Design review of the part built by this model. Coordinates are the model's own, in mm. A direction names the side the tool comes from. Coordinates: 2 decimals unless noted, no trailing zeros. Write each loop counter-clockwise with the first axis right and the second up, starting at its lowest first coordinate (ties: lowest second). Pieces come first, ordered by that corner, then holes.
Q1. For faces 1 (the cylindrical face through (-15.02, 3.23, 0.53)), 2 (the flat face through (9.01, 3.51, -1.74)), 3 (the flat face through (-13.01, 0.99, -1.74)), list the 3-axis set-ups (+Z, -Z, +X, -X, +Y, -Y) from which the entire face can be reached by the end or side of a thin tool; tool diameter is ignored.
Q2. Take a section at B-B, the plane y = 2.9. Write out the cut boundary in (x, z).
Q3. The part is to be moulded in two halves that separate along Z. For faces 4 (the flat face through (-12, 1, 0)), 5 (the flat face through (-5, 4.5, 5)), 6 (the cylindrical face through (-17.46, 2.22, -0.52)), say which applies: released by +Z, released by -Z, zero draft, split by the parting line, or undercut.
Q4. For pin 1 Ø0.6 at (y, z) = (1, -0.5) entering from -X; pin 2 Ø1.2 at (x, z) = (9.5, 0.5) entering from +Y; pin 3 Ø1 at (y, z) = (2.5, 8) entering from +X, all flat-tipped, find the tip position at first contact; note any pin that passes through.
Q5. For L1, parallel to X at y = 1.6, z = 0; L2, parallel to X at y = 0.35, z = 0; L3, parallel to X at y = 3, z = -2.25, list the stretches that pass through material, from the lowest coordinate up.
Q6. Take a section at D-D, the plane x = -10.5. Write out the cut boundary in (y, z).
Q7. Take a section at C-C, the plane x = 0. Write out the cut boundary in (y, z), plus the area to 4 significant figures.
Q8. Take a section at A-A, the plane z = 0. Write out the cut boundary in (x, y), plus the area to 3 significant figures.
from build123d import *

# Parameters (mm, degrees)
SKETCH1_R           = 4
SKETCH1_R_2         = 1.15
BOSS_EXTRUDE1_DEPTH = 4.5
SKETCH2_R           = 6
CUT_EXTRUDE1_DEPTH  = 3.5
CUT_EXTRUDE2_DEPTH  = 2
CUT_EXTRUDE3_DEPTH  = 2


with BuildPart() as part:
    # Sketch1 → Boss-Extrude1 (new body)
    with BuildSketch(Plane(origin=(0, 0, 0), x_dir=(1, 0, 0), z_dir=(0, 1, 0))):
        with BuildLine():
            Line((3, 6.873863542), (11.4, 3.207802986))
            ThreePointArc((11.4, 3.207802986), (13.439020979, 0.650488054), (12.474873734, -2.474873734))
            Line((12.474873734, -2.474873734), (2.474873734, -12.474873734))
            ThreePointArc((2.474873734, -12.474873734), (0.28868186, -13.488074366), (-2.034333678, -12.848067149))
            Line((-2.034333678, -12.848067149), (-16.034333678, -2.848067149))
            ThreePointArc((-16.034333678, -2.848067149), (-17.452321053, 0.575742432), (-15, 3.354101966))
            Line((-15, 3.354101966), (-2.142857143, 7.187361356))
            ThreePointArc((-2.142857143, 7.187361356), (0.456337254, 7.486104215), (3, 6.873863542))
        make_face()
        with Locations(Location((0, 0, 0), (0, 0, 270))):
            Circle(SKETCH1_R, mode=Mode.SUBTRACT)
        with Locations(Location((-14, 0, 0), (0, 0, 270))):
            Circle(SKETCH1_R_2, mode=Mode.SUBTRACT)
        with Locations(Location((10, 0, 0), (0, 0, 270))):
            Circle(SKETCH1_R_2, mode=Mode.SUBTRACT)
        with Locations(Location((0, -10, 0), (0, 0, 270))):
            Circle(SKETCH1_R_2, mode=Mode.SUBTRACT)
    extrude(amount=BOSS_EXTRUDE1_DEPTH)

    # Sketch2 → Cut-Extrude1 (cut)
    with BuildSketch(Plane(origin=(0, 4.5, 0), x_dir=(1, 0, 0), z_dir=(0, 1, 0))):
        with Locations(Location((0, 0, 0), (0, 0, 270))):
            Circle(SKETCH2_R)
    extrude(amount=-CUT_EXTRUDE1_DEPTH, mode=Mode.SUBTRACT)

    # Sketch3 → Cut-Extrude2 (cut)
    with BuildSketch(Plane(origin=(0, 4.5, 0), x_dir=(1, 0, 0), z_dir=(0, 1, 0))):
        Polygon((12, -1.154700538), (12, 1.154700538), (10, 2.309401077), (8, 1.154700538), (8, -1.154700538), (10, -2.309401077), align=None)
        Polygon((2.309401077, -10), (1.154700538, -8), (-1.154700538, -8), (-2.309401077, -10), (-1.154700538, -12), (1.154700538, -12), align=None)
    extrude(amount=-CUT_EXTRUDE2_DEPTH, mode=Mode.SUBTRACT)

    # Sketch4 → Cut-Extrude3 (cut)
    with BuildSketch(Plane.XZ):
        Polygon((-12, -1.154700538), (-12, 1.154700538), (-14, 2.309401077), (-16, 1.154700538), (-16, -1.154700538), (-14, -2.309401077), align=None)
    extrude(amount=-CUT_EXTRUDE3_DEPTH, mode=Mode.SUBTRACT)


solid = part.part
Responses:
1. face 1: +Y, -Y
1. face 2: +Y
1. face 3: -Y
2. outline: (-16.03, 2.85) arc R3.5 ccw to (-15, -3.35) - (-2.14, -7.19) arc R7.5 ccw to (3, -6.87) - (11.4, -3.21) arc R3.5 ccw to (12.47, 2.47) - (2.47, 12.47) arc R3.5 ccw to (-2.03, 12.85) - close; hole circle Ø2.3 at (-14, 0); hole circle Ø12 at (0, 0); hole (-2.31, 10) - (-1.15, 8) - (1.15, 8) - (2.31, 10) - (1.15, 12) - (-1.15, 12) - close; hole (8, -1.15) - (10, -2.31) - (12, -1.15) - (12, 1.15) - (10, 2.31) - (8, 1.15) - close
3. face 4: undercut
3. face 5: zero draft
3. face 6: split by the parting line
4. pin 1: stops at x = -17.49
4. pin 2: stops at y = 2.5
4. pin 3: stops at x = 7.45
5. L1: x = -17.5 to -16, -12 to -6, 6 to 8.85, 11.15 to 13.5
5. L2: x = -17.5 to -16, -12 to -4, 4 to 8.85, 11.15 to 13.5
5. L3: x = -16.68 to -5.56, 5.56 to 9.9, 10.1 to 12.68
6. outline: (0, -4.7) - (4.5, -4.7) - (4.5, 6.8) - (0, 6.8) - close
7. outline: (0, -7.5) - (4.5, -7.5) - (4.5, -6) - (1, -6) - (1, -4) - (0, -4) - close; (0, 4) - (1, 4) - (1, 6) - (4.5, 6) - (4.5, 8) - (2.5, 8) - (2.5, 8.85) - (0, 8.85) - close; (0, 11.15) - (2.5, 11.15) - (2.5, 12) - (4.5, 12) - (4.5, 13.5) - (0, 13.5) - close
7. area: 30.75 mm2
8. outline: (-17.5, 0) - (-16, 0) - (-16, 2) - (-15.15, 2) - (-15.15, 4.5) - (-17.5, 4.5) - close; (-12.85, 2) - (-12, 2) - (-12, 0) - (-4, 0) - (-4, 1) - (-6, 1) - (-6, 4.5) - (-12.85, 4.5) - close; (4, 0) - (8.85, 0) - (8.85, 2.5) - (8, 2.5) - (8, 4.5) - (6, 4.5) - (6, 1) - (4, 1) - close; (11.15, 0) - (13.5, 0) - (13.5, 4.5) - (12, 4.5) - (12, 2.5) - (11.15, 2.5) - close
8. area: 62.0 mm2
